```python
from build123d import *

# Parameters (mm, degrees)
BOSS_EXTRUDE1_DEPTH      = 10
BOSS_EXTRUDE2_DEPTH      = 5
BOSS_EXTRUDE2_DEPTH_BACK = 5
SKETCH3_R                = 11
BOSS_EXTRUDE3_DEPTH      = 13.9
BOSS_EXTRUDE3_DEPTH_BACK = 13.9
SKETCH4_W                = 3.3
SKETCH4_H                = 10
SKETCH5_W                = 3.3
SKETCH5_H                = 10
SKETCH6_W                = 3.3
SKETCH6_H                = 10
SKETCH7_W                = 3.3
SKETCH7_H                = 10


with BuildPart() as part:
    # Sketch1 → Boss-Extrude1 (new body)
    with BuildSketch(Plane(origin=(0, 0, 0), x_dir=(1, 0, 0), z_dir=(0, 1, 0))):
        with BuildLine():
            Line((-21, -17.5), (21, -17.5))
            ThreePointArc((21, -17.5), (25.242640687, -15.742640687), (27, -11.5))
            Line((27, -11.5), (27, 11.5))
            ThreePointArc((27, 11.5), (25.242640687, 15.742640687), (21, 17.5))
            Line((21, 17.5), (-21, 17.5))
            ThreePointArc((-21, 17.5), (-25.242640687, 15.742640687), (-27, 11.5))
            Line((-27, 11.5), (-27, -11.5))
            ThreePointArc((-27, -11.5), (-25.242640687, -15.742640687), (-21, -17.5))
        make_face()
    extrude(amount=BOSS_EXTRUDE1_DEPTH)

    # Sketch2 → Boss-Extrude2 (add, two sides)
    with BuildSketch(Plane(origin=(0, 0, 0), x_dir=(0, 0, -1), z_dir=(1, 0, 0))) as boss_extrude2_sk:
        Polygon((-23.698557159, 33.133330249), (-17.5, 10), (14.884597423, 10), (-3.630389444, 38.510579582), align=None)
    extrude(amount=BOSS_EXTRUDE2_DEPTH)
    extrude(boss_extrude2_sk.sketch, amount=-BOSS_EXTRUDE2_DEPTH_BACK)

    # Sketch3 → Boss-Extrude3 (add, two sides)
    with BuildSketch(Plane(origin=(0, 0, 0), x_dir=(0, 0, -1), z_dir=(1, 0, 0))) as boss_extrude3_sk:
        with Locations((-13, 36)):
            Circle(SKETCH3_R)
    extrude(amount=BOSS_EXTRUDE3_DEPTH)
    extrude(boss_extrude3_sk.sketch, amount=-BOSS_EXTRUDE3_DEPTH_BACK)

    # Sketch4 → Cut-Revolve1 (revolve, cut)
    with BuildSketch(Plane.XY.offset(11)):
        with Locations((-22.15, 5)):
            Rectangle(SKETCH4_W, SKETCH4_H)
    revolve(axis=Axis((-20.5, 10, 11), (0, -1, 0)), mode=Mode.SUBTRACT)

    # Sketch5 → Cut-Revolve2 (revolve, cut)
    with BuildSketch(Plane.XY.offset(11)):
        with Locations((18.85, 5)):
            Rectangle(SKETCH5_W, SKETCH5_H)
    revolve(axis=Axis((20.5, 10, 11), (0, -1, 0)), mode=Mode.SUBTRACT)

    # Sketch6 → Cut-Revolve3 (revolve, cut)
    with BuildSketch(Plane.XY.offset(-11)):
        with Locations((-22.15, 5)):
            Rectangle(SKETCH6_W, SKETCH6_H)
    revolve(axis=Axis((-20.5, 10, -11), (0, -1, 0)), mode=Mode.SUBTRACT)

    # Sketch7 → Cut-Revolve4 (revolve, cut)
    with BuildSketch(Plane.XY.offset(-11)):
        with Locations((18.85, 5)):
            Rectangle(SKETCH7_W, SKETCH7_H)
    revolve(axis=Axis((20.5, 10, -11), (0, -1, 0)), mode=Mode.SUBTRACT)

    # Sketch8 → Cut-Revolve5 (revolve, cut)
    with BuildSketch(Plane.XY.offset(13)):
        Polygon((-13.9, 36), (-13.9, 45.5), (-13.611324865, 45), (13.611324865, 45), (13.9, 45.5), (13.9, 36), align=None)
    revolve(axis=Axis((13.9, 36, 13), (-1, 0, 0)), mode=Mode.SUBTRACT)

    # Sketch9 → Revolve1 (revolve)
    with BuildSketch(Plane.XY.offset(13)):
        Polygon((-13.9, 42.3), (-13.6, 42), (13.6, 42), (13.9, 42.3), (13.9, 44.7), (13.6, 45), (-13.6, 45), (-13.9, 44.7), align=None)
    revolve(axis=Axis((13.9, 36, 13), (-1, 0, 0)))


solid = part.part
```
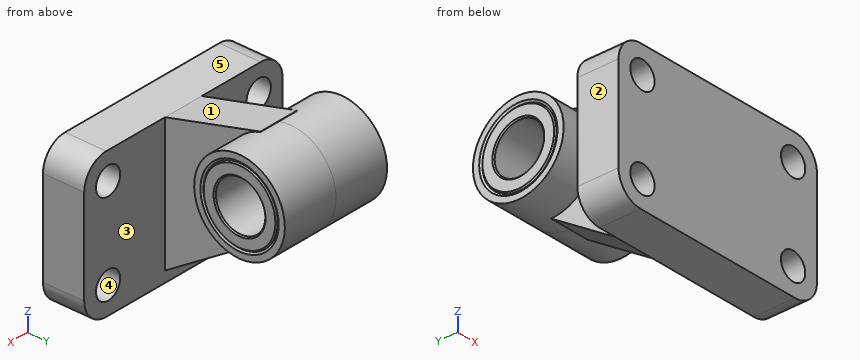
The listing builds one solid part. Answer for the finished solid, in the listing's coordinates (mm). Face numbers are marked on the shaded views. A direction names the side the tool comes from. Coordinates: 2 decimals unless noted, no trailing zeros. Loops run counter-clockwise (first coordinate to the right, second up) from the corner with the lowest first, then second, coordinate; pieces in that order, holes last. Notation, with made-up numbers: M 8,72.25 L 36,72.25 A20 ccw 36,104.25 Z; hole C 55,1.5 d4. An arc over 180 degrees is marked long. Answer as CSV lines item,"result". Start each with the question number.
(1) Find the intervals of material crossed by L1, parallel to Z at x = -13.55, y = 36; L2, parallel to Z at x = 20.5, y = 3; L3, parallel to Z at x = -22, y = 9, in increasing order. Write a range as [from, to].
(2) The part is cut by section B-B (x = -2). Give the vertices of the cut face in (y, z), and give its area (3 significant figures).
(3) Given pin 1 (17.5 mm diameter, centred on y = 34, z = 11, fed in from +X); pin 2 (8.5 mm diameter, centred on y = 39, z = 11, fed in from -X); pin 3 (4 mm diameter, centred on x = -15.5, y = 40.5, fed in from +Z), each flat-ended and moving along its own axis, determine where each tip first touches the part or whether it passes through.
(4) The part is cut by section A-A (x = -10.5). Give the vertices of the cut face in (y, z), and give its area (3 significant figures).
(5) For the marked faces 4 and 5, determine the directions among +Z, -Z, +X, -X, +Y, -Y from which every point of the face is accessible in a straight line to the end or side of a thin tool.
(6) The mould has two halves that part along Y. Classify the marked faces 1, 2 and 3: pulls with the +Y half, pulls with the -Y half, needs draft (parallel to the pull), parting line crosses it, or undercut.
(7) The part is cut by section D-D (z = 13). State how many separate pieces and enclosed holes the cut face has, and give its area (3 significant figures).
(8) The part is cut by section C-C (x = -18.5). Give the vertices of the cut face in (y, z), and give its area (3 significant figures).
Determined:
1,L1,"[2, 7], [19, 24]"
1,L2,"[-17.5, -14.3], [-7.7, 7.7], [14.3, 17.5]"
1,L3,"[-17.42, -13.94], [-8.06, 8.06], [13.94, 17.42]"
2,outline,"M 0,-17.5 L 10,-17.5 L 10,-14.88 L 36,2 A11 ccw long 33.15,23.63 L 33.13,23.7 L 10,17.5 L 0,17.5 Z; hole C 36,13 d12"
2,area,"1,140 mm2"
3,pin 1,"x = 13.9"
3,pin 2,"x = -13.9"
3,pin 3,"z = 23.49"
4,outline,"M 0,-17.5 L 10,-17.5 L 10,17.5 L 0,17.5 Z; C 36,13 d22; hole C 36,13 d12"
4,area,"617 mm2"
5,face 4,"+Y, -Y"
5,face 5,"+Z, +X, -X, -Y"
6,face 1,"pulls with the -Y half"
6,face 2,"needs draft"
6,face 3,"undercut"
7,separate pieces,"4"
7,enclosed holes,"0"
7,area,"859 mm2"
8,outline,"M 0,-17.5 L 10,-17.5 L 10,-13.62 L 0,-13.62 Z; M 0,-8.38 L 10,-8.38 L 10,8.38 L 0,8.38 Z; M 0,13.62 L 10,13.62 L 10,17.5 L 0,17.5 Z"
8,area,"245 mm2"
